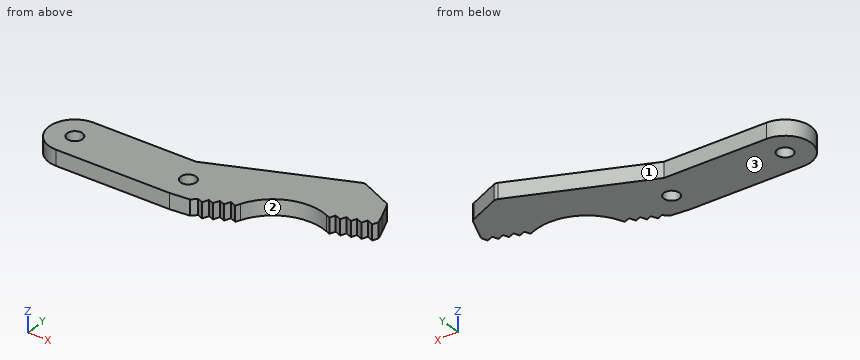
```python
from build123d import *

# Parameters (mm, degrees)
SKETCH1_R           = 1.5
BOSS_EXTRUDE1_DEPTH = 3


with BuildPart() as part:
    # Sketch1 → Boss-Extrude1 (new body)
    with BuildSketch(Plane.XY):
        with BuildLine():
            Line((0, 5), (19.85, 5))
            Line((19.85, 5), (44.643069029, 15.193663072))
            ThreePointArc((44.643069029, 15.193663072), (45.042006379, 15.268610471), (45.43786686, 15.178818479))
            Line((45.43786686, 15.178818479), (51.245085043, 12.533540635))
            ThreePointArc((51.245085043, 12.533540635), (51.550738574, 12.317286013), (51.755428853, 12.003770413))
            Line((51.755428853, 12.003770413), (52.954960556, 9.086264498))
            Line((52.954960556, 9.086264498), (53.647413738, 7.201821951))
            Line((53.647413738, 7.201821951), (53.200417763, 6.109762155))
            Line((53.200417763, 6.109762155), (51.987413738, 6.606262365))
            Line((51.987413738, 6.606262365), (51.540417763, 5.514202569))
            Line((51.540417763, 5.514202569), (50.327413738, 6.010702778))
            Line((50.327413738, 6.010702778), (49.901790908, 4.970859901))
            Line((49.901790908, 4.970859901), (48.688786884, 5.467360111))
            Line((48.688786884, 5.467360111), (48.241790908, 4.375300315))
            Line((48.241790908, 4.375300315), (47.028786884, 4.871800524))
            Line((47.028786884, 4.871800524), (46.581790908, 3.779740729))
            Line((46.581790908, 3.779740729), (45.736822648, 4.125598541))
            ThreePointArc((45.736822648, 4.125598541), (38.240209852, 4.168619257), (32.907533275, -1.100499713))
            Line((32.907533275, -1.100499713), (32.521118505, -2.009071771))
            Line((32.521118505, -2.009071771), (31.373673566, -1.521064608))
            Line((31.373673566, -1.521064608), (30.860706561, -2.727197301))
            Line((30.860706561, -2.727197301), (29.774832981, -2.265376374))
            Line((29.774832981, -2.265376374), (29.261865976, -3.471509067))
            Line((29.261865976, -3.471509067), (28.227913521, -3.031770141))
            Line((28.227913521, -3.031770141), (27.714946516, -4.237902834))
            Line((27.714946516, -4.237902834), (26.629072936, -3.776081907))
            Line((26.629072936, -3.776081907), (25.729131342, -4.679393535))
            Line((25.729131342, -4.679393535), (22, -5))
            Line((22, -5), (0, -5))
            ThreePointArc((0, -5), (-5, 0), (0, 5))
        make_face()
        Circle(SKETCH1_R, mode=Mode.SUBTRACT)
        with Locations((22, 0)):
            Circle(SKETCH1_R, mode=Mode.SUBTRACT)
    extrude(amount=BOSS_EXTRUDE1_DEPTH)


solid = part.part
```
Can you work these out from the model? Positions are in its coordinate system, mm. Face numbers are marked on the shaded views. Coordinates: 2 decimals unless noted, no trailing zeros. Order: outer loops, then holes, each group sorted by start corner. A loop starts at its lowest first (then second) coordinate and runs counter-clockwise, first axis right, second up. Notation, with made-up numbers: (48.5, 66.5) - (53.5, 66.5) arc R31 cw to (53.5, 91.5) - close; hole circle Ø6 at (39, 37). An arc over 180 degrees is marked (long way). Answer in a Markdown table with one row per item.
1. Suppose I cut it at D-D (y = 3.25). Please give me the cut outline in (x, z), and give its area (3 significant figures).
Reply:
| item | result |
|---|---|
| outline | (-3.8, 0) - (36.51, 0) - (36.51, 3) - (-3.8, 3) - close |
| area | 121 mm^2 |
2. For pin 1 (2.5 mm diameter, centred on x = 22, y = 0, fed in from +Z); pin 2 (3.5 mm diameter, centred on x = 0, y = 0, fed in from -Z); pin 3 (1.5 mm diameter, centred on x = 6.5, z = 1.5, fed in from +Y), each with a flat end and sliding along its axis, tell me the tip position at first contact or that it passes through.
Reply:
| item | result |
|---|---|
| pin 1 | passes through |
| pin 2 | stops at z = 0 |
| pin 3 | stops at y = 5 |
3. Suppose I cut it at B-B (y = 0). Please give me the cut outline in (x, z).
Reply:
| item | result |
|---|---|
| outline | (-5, 0) - (-1.5, 0) - (-1.5, 3) - (-5, 3) - close; (1.5, 0) - (20.5, 0) - (20.5, 3) - (1.5, 3) - close; (23.5, 0) - (33.45, 0) - (33.45, 3) - (23.5, 3) - close |
4. If we mould it in two halves opening along X, with no side actions, what happens to the marked faces 1, 2 and 3? For each: pulls with the +X half, pulls with the -X half, needs draft (parallel to the pull), parting line crosses it, or undercut.
Reply:
| item | result |
|---|---|
| face 1 | pulls with the -X half |
| face 2 | undercut |
| face 3 | needs draft |
5. If I drill on line 1 along Y through (x, z) = (0, 1.35); line 2 along Y through (x, z) = (3, 1.5); line 3 along X through (y, z) = (-0.25, 1.65), over which ranges is the centre line in solid material (lowest first)?
Reply:
| item | result |
|---|---|
| line 1 | y = -5 to -1.5, 1.5 to 5 |
| line 2 | y = -5 to 5 |
| line 3 | x = -4.99 to -1.48, 1.48 to 20.52, 23.48 to 33.32 |
6. Suppose I cut it at C-C (x = 12). Please give me the cut outline in (y, z), and give its area (3 significant figures).
Reply:
| item | result |
|---|---|
| outline | (-5, 0) - (5, 0) - (5, 3) - (-5, 3) - close |
| area | 30.0 mm^2 |
7. Suppose I cut it at A-A (z = 0.45). Give the number of separate pieces and of enclosed holes in the cut face, and give its area (3 significant figures).
Reply:
| item | result |
|---|---|
| separate pieces | 1 |
| enclosed holes | 2 |
| area | 552 mm^2 |
